The figure shows three views and two pictorial views of one solid part (mm, origin at its lowest corner). Answer the questions. A direction names the side the tool comes from. Coordinates: 2 decimals unless noted, no trailing zeros. Order: outer loops, then holes, each group sorted by start corner. A loop starts at its lowest first (then second) coordinate and runs counter-clockwise, first axis right, second up. Notation, with made-up numbers: (24.5, 42) -> (70.5, 42) arc R11 ccw to (70.5, 55) -> close; hole circle Ø5 at (62, 24). An arc over 180 degrees is marked (long way). Return JSON: item names as keys, results as strings.
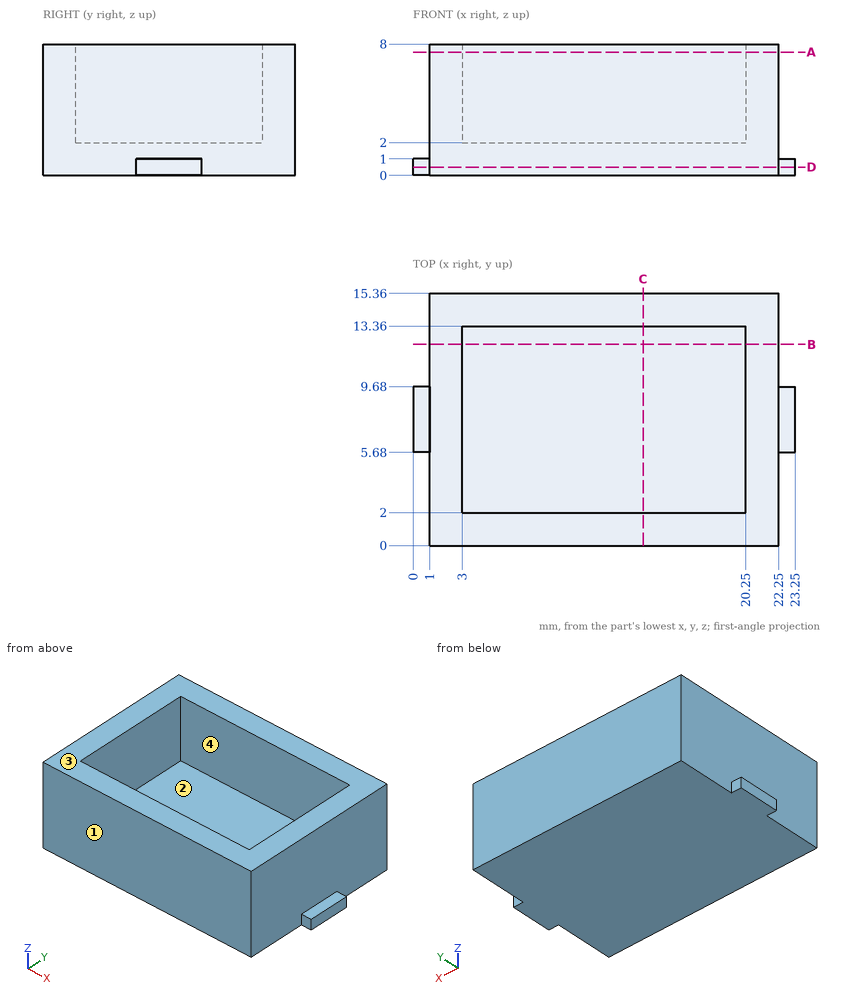
Item 1: The part is cut by section B-B on y = 12.25. Determine the outline of the cut face in (x, z), plus the area to 3 significant figures.
Answer list:
{"outline": "(1, 0) -> (22.25, 0) -> (22.25, 8) -> (20.25, 8) -> (20.25, 2) -> (3, 2) -> (3, 8) -> (1, 8) -> close", "area": "66.5 mm2"}
Item 2: Find the intervals of material crossed by probe 1 along Y at (x, z) = (4, 6); probe 2 along X at (y, z) = (12, 4.25); probe 3 along Z at (x, y) = (15, 9.25), in increasing order.
Answer list:
{"probe 1": "0 to 2, 13.36 to 15.36", "probe 2": "1 to 3, 20.25 to 22.25", "probe 3": "0 to 2"}
Item 3: Which of the six approach directions +Z, -Z, +X, -X, +Y, -Y give full straight-line access (tool end or side, diameter ignored) to the marked faces 3 and 4?
Answer list:
{"face 3": "+Z, +X, -X, +Y, -Y", "face 4": "+Z"}
Item 4: The part is cut by section D-D on z = 0.5. Determine the outline of the cut face in (x, y).
Answer list:
{"outline": "(0, 5.68) -> (1, 5.68) -> (1, 0) -> (22.25, 0) -> (22.25, 5.68) -> (23.25, 5.68) -> (23.25, 9.68) -> (22.25, 9.68) -> (22.25, 15.36) -> (1, 15.36) -> (1, 9.68) -> (0, 9.68) -> close"}
Item 5: Flat-ended cylindrical pins translate along their axes: pin 1 (0.5 mm diameter, centred on x = 23, z = 0.5, fed in from -Y); pin 2 (4 mm diameter, centred on y = 10.5, z = 5, fed in from +X); pin 3 (1.8 mm diameter, centred on y = 8, z = 6, fed in from -X). Find the tip coordinate at first contact, or state that the pin passes through.
Answer list:
{"pin 1": "y = 5.68", "pin 2": "x = 22.25", "pin 3": "x = 1"}
Item 6: Determine the mould class of the marked faces 1 and 2 for opening direction X: pulls with the +X half, pulls with the -X half, needs draft (parallel to the pull), parting line crosses it, or undercut.
Answer list:
{"face 1": "needs draft", "face 2": "undercut"}
Item 7: The part is cut by section C-C on x = 14. Determine the outline of the cut face in (y, z), plus the area to 3 significant figures.
Answer list:
{"outline": "(0, 0) -> (15.36, 0) -> (15.36, 8) -> (13.36, 8) -> (13.36, 2) -> (2, 2) -> (2, 8) -> (0, 8) -> close", "area": "54.7 mm2"}
Item 8: The part is cut by section A-A on z = 7.5. Determine the outline of the cut face in (x, y), plus the area to 3 significant figures.
Answer list:
{"outline": "(1, 0) -> (22.25, 0) -> (22.25, 15.36) -> (1, 15.36) -> close; hole (3, 2) -> (20.25, 2) -> (20.25, 13.36) -> (3, 13.36) -> close", "area": "130 mm2"}
